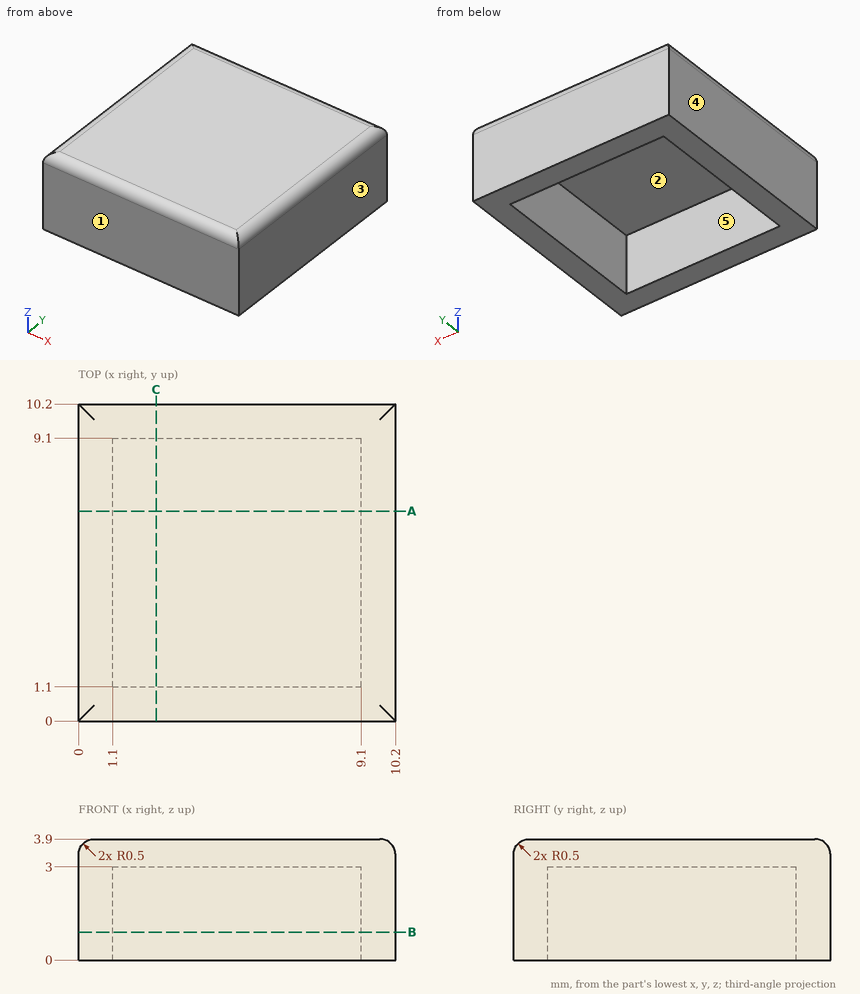
Design review of the part shown in the three views and the two pictorial views. Dimensions are in mm from the part's minimum x, y and z. A direction names the side the tool comes from. Round coordinates to 2 decimals unless told otherwise and drop trailing zeros. Loops run counter-clockwise (first coordinate to the right, second up) from the corner with the lowest first, then second, coordinate; pieces in that order, holes last.
Q1. To check wall thickness, follow line 1 along Y through (x, z) = (4, 2.1); line 2 along Z through (x, y) = (7.5, 8.25). State the ranges of each line that lie inside material, in increasing order.
Result sheet:
line 1: y = 0 to 1.1, 9.1 to 10.2
line 2: z = 3 to 3.9
Q2. Machinability: for the marked faces 4 and 5, which of the approach directions +Z, -Z, +X, -X, +Y, -Y give a long, thin tool a straight path to every point of the face, cutting with its end or side? Answer none if there is none.
Result sheet:
face 4: +Z, -Z, -X, +Y, -Y
face 5: -Z
Q3. Add section A-A on y = 6.75. Write out the cut boundary in (x, z), plus the area to 3 significant figures.
Result sheet:
outline: (0, 0) - (1.1, 0) - (1.1, 3) - (9.1, 3) - (9.1, 0) - (10.2, 0) - (10.2, 3.4) arc R0.5 ccw to (9.7, 3.9) - (0.5, 3.9) arc R0.5 ccw to (0, 3.4) - close
area: 15.7 mm2
Q4. Insertion check: pin 1 Ø4 at (x, y) = (5.5, 5) entering from -Z; pin 2 Ø1.5 at (x, z) = (5.5, 2) entering from -Y. Each pin has a flat end and moves straight along its axis. Give the tip position at first contact, or say it passes through.
Result sheet:
pin 1: stops at z = 3
pin 2: stops at y = 0
Q5. Mouldability with a two-part tool opening along Y and no side actions: class the marked faces 1, 2 and 3 as +Y half, -Y half, draft (parallel to the pull), parting line (faces both ways), or undercut.
Result sheet:
face 1: -Y half
face 2: undercut
face 3: draft
Q6. Add section B-B on z = 0.9. Write out the cut boundary in (x, y).
Result sheet:
outline: (0, 0) - (10.2, 0) - (10.2, 10.2) - (0, 10.2) - close; hole (1.1, 1.1) - (9.1, 1.1) - (9.1, 9.1) - (1.1, 9.1) - close
